```python
from build123d import *

# Parameters (mm, degrees)
F0_R     = 20
F0_R_2   = 13
F1_DEPTH = 3
F2_R     = 15
F2_R_2   = 13
F3_DEPTH = 20
F4_R     = 2.5
F5_SIZE2 = 4
F5_SIZE  = 0.75


# Not quite as in the source:
# - a fillet or chamfer that OpenCascade refuses, or shapes differently, is made with other operations: its cross-section is extruded or revolved along the edge and cut away or added


with BuildPart() as f1:
    # F0 (on Top) → F1 (new body)
    with BuildSketch(Plane.XY):
        Circle(F0_R)
        Circle(F0_R_2, mode=Mode.SUBTRACT)
    extrude(amount=F1_DEPTH)

    # F2 (on face) → F3 (join)
    with BuildSketch(Plane.XY.offset(3)):
        Circle(F2_R)
        Circle(F2_R_2, mode=Mode.SUBTRACT)
    extrude(amount=F3_DEPTH)

    # F4
    f4_edges = [f1.edges().sort_by_distance(p)[0] for p in [
        (-20, 0, 3),
    ]]
    fillet(f4_edges, radius=F4_R)

    # F5
    f5_edges = [f1.edges().sort_by_distance(p)[0] for p in [
        (-13, 0, 23),
    ]]
    f5_side = f1.faces().sort_by_distance((-14.575736, 0, 23))[0]
    chamfer(f5_edges, length=F5_SIZE, length2=F5_SIZE2, reference=f5_side)

    # F6: fillet of radius 2 on 1 edges, made by hand

    # F6_s1 → F6_t2 (revolve, cut)
    with BuildSketch(Plane.XZ):
        with BuildLine():
            ThreePointArc((13.75, 23), (14.6583123952, 22.263984367), (15, 21.1459503782))
            Line((15, 21.1459503782), (15, 23))
            Line((15, 23), (13.75, 23))
        make_face()
    revolve(axis=Axis((0, 0, 23), (0, 0, 1)), mode=Mode.SUBTRACT)


solid = f1.part
```
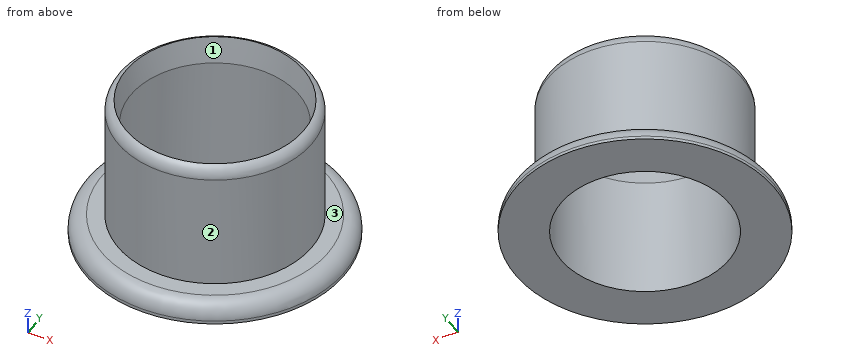
Here's how the part is built. I have some questions about the finished solid (model axes, mm). Face numbers are marked on the shaded views. Coordinates: 2 decimals unless noted, no trailing zeros. Loops run counter-clockwise (first coordinate to the right, second up) from the corner with the lowest first, then second, coordinate; pieces in that order, holes last. Notation, with made-up numbers: (55, 42.5) -> (74, 42.5) arc R15 cw to (74, 65.5) -> close; hole circle Ø11 at (5, 77). An arc over 180 degrees is marked (long way). Return JSON: item names as keys, results as strings.
1) I need wall thicknesses on line 1 (Y direction, x = 0, z = 10); line 2 (Y direction, x = 9.5, z = 20); line 3 (X direction, y = -1.5, z = 8). Which ranges of each line are inside material? Lowest first, please. Write a range as from..to.
Results below:
{"line 1": "-15..-13, 13..15", "line 2": "-11.61..-9.15, 9.15..11.61", "line 3": "-14.92..-12.91, 12.91..14.92"}
2) If we section it at A-A, the plane y = 0: Write out the boundary of the cut face in (x, z), then the cut area to 3 significant figures.
Results below:
{"outline": "(-20, 0) -> (-13, 0) -> (-13, 19) -> (-13.75, 23) arc R2 ccw to (-15, 21.15) -> (-15, 3) -> (-17.5, 3) arc R2.5 ccw to (-20, 0.5) -> close; (13, 0) -> (20, 0) -> (20, 0.5) arc R2.5 ccw to (17.5, 3) -> (15, 3) -> (15, 21.15) arc R2 ccw to (13.75, 23) -> (13, 19) -> close", "area": "115 mm²"}
3) Thinking about a two-plate mould opening in Y: for the marked faces 1, 2 and 3, which applies, +Y half, -Y half, draft (parallel to the pull), parting line (faces both ways), or undercut?
Results below:
{"face 1": "undercut", "face 2": "parting line", "face 3": "draft"}
4) If we section it at C-C, the plane z = 15.5: Write out the boundary of the cut face in (x, y).
Results below:
{"outline": "circle Ø30 at (0, 0); hole circle Ø26 at (0, 0)"}
5) If we section it at D-D, the plane z = 2.25: Write out the boundary of the cut face in (x, y), then the cut area to 3 significant figures.
Results below:
{"outline": "circle Ø38.57 at (0, 0); hole circle Ø26 at (0, 0)", "area": "638 mm²"}
6) Will these pins go through, and if not, where does the flat tip stop? pin 1 (2 mm diameter, centred on y = -11.5, z = 19, fed in from +X); pin 2 (1.5 mm diameter, centred on y = -4.5, z = 17.5, fed in from +X); pin 3 (1.5 mm diameter, centred on x = -1.5, z = 2.5, fed in from -Y).
Results below:
{"pin 1": "x = 10.71", "pin 2": "x = 14.52", "pin 3": "y = -19.61"}
